Model file for the job. Use its own axes, mm. Coordinates: 2 decimals unless noted, no trailing zeros. Loops run counter-clockwise (first coordinate to the right, second up) from the corner with the lowest first, then second, coordinate; pieces in that order, holes last.
from build123d import *

# Parameters (mm, degrees)
SKETCH1_R           = 80
BOSS_EXTRUDE1_DEPTH = 20
SKETCH3_R           = 15
BOSS_EXTRUDE2_DEPTH = 15
CHAMFER1_SIZE       = 5
FILLET2_R           = 5
FILLET3_R           = 5
SKETCH4_R           = 5
CUT_EXTRUDE2_DEPTH  = 20


with BuildPart() as part:
    # Sketch1 → Boss-Extrude1 (new body)
    with BuildSketch(Plane(origin=(0, 0, 0), x_dir=(1, 0, 0), z_dir=(0, 1, 0))):
        with Locations(Location((-29.715512057, 28.347034528, 0), (0, 0, 270))):
            Circle(SKETCH1_R)
    extrude(amount=BOSS_EXTRUDE1_DEPTH)

    # Sketch3 → Boss-Extrude2 (add)
    with BuildSketch(Plane(origin=(0, 20, 0), x_dir=(1, 0, 0), z_dir=(0, 1, 0))):
        with Locations(Location((-29.715512057, 28.347034528, 0), (0, 0, 270))):
            Circle(SKETCH3_R)
    extrude(amount=BOSS_EXTRUDE2_DEPTH)

    # Chamfer1
    chamfer1_edges = [part.edges().sort_by_distance(p)[0] for p in [
        (-29.715512057, 35, -43.347034528),
    ]]
    chamfer(chamfer1_edges, length=CHAMFER1_SIZE)

    # Fillet2
    fillet2_edges = [part.edges().sort_by_distance(p)[0] for p in [
        (-29.715512057, 20, -108.347034528),
    ]]
    fillet(fillet2_edges, radius=FILLET2_R)

    # Fillet3
    fillet3_edges = [part.edges().sort_by_distance(p)[0] for p in [
        (-29.715512057, 0, -108.347034528),
    ]]
    fillet(fillet3_edges, radius=FILLET3_R)

    # Sketch4 → Cut-Extrude2 (cut)
    with BuildSketch(Plane(origin=(0, 20, 0), x_dir=(1, 0, 0), z_dir=(0, 1, 0))):
        with Locations(Location((-29.715512057, 77.081261822, 0), (0, 0, 270))):
            Circle(SKETCH4_R)
        with Locations(Location((-1.070251971, 67.773852617, 0), (0, 0, 270))):
            Circle(SKETCH4_R)
        with Locations(Location((16.633492378, 43.406738969, 0), (0, 0, 270))):
            Circle(SKETCH4_R)
        with Locations(Location((16.633492378, 13.287330086, 0), (0, 0, 270))):
            Circle(SKETCH4_R)
        with Locations(Location((-1.070251971, -11.079783561, 0), (0, 0, 270))):
            Circle(SKETCH4_R)
        with Locations(Location((-29.715512057, -20.387192767, 0), (0, 0, 270))):
            Circle(SKETCH4_R)
        with Locations(Location((-58.360772142, -11.079783561, 0), (0, 0, 270))):
            Circle(SKETCH4_R)
        with Locations(Location((-76.064516492, 13.287330086, 0), (0, 0, 270))):
            Circle(SKETCH4_R)
        with Locations(Location((-76.064516492, 43.406738969, 0), (0, 0, 270))):
            Circle(SKETCH4_R)
        with Locations(Location((-58.360772142, 67.773852617, 0), (0, 0, 270))):
            Circle(SKETCH4_R)
    extrude(amount=-CUT_EXTRUDE2_DEPTH, mode=Mode.SUBTRACT)


solid = part.part
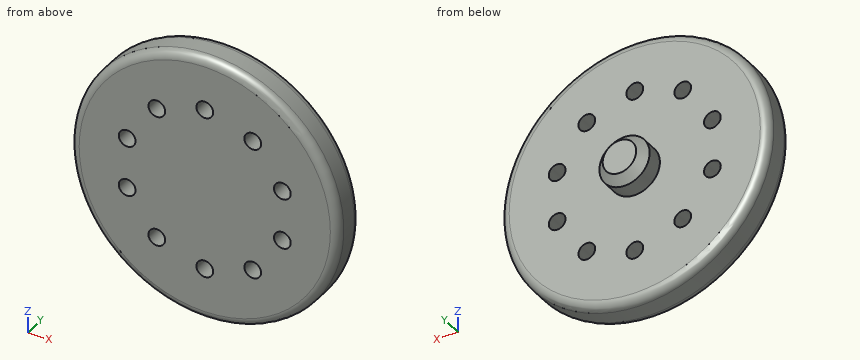
Q1. Flat gauge pins, fed straight in: P1, Ø8, axis at x = -78.5, y = 8, coming from the +Z side; P2, Ø6, axis at x = 5, y = 18, coming from the +Z side; P3, Ø12, axis at x = 31, y = 15, coming from the +Z side. Where does each tip first touch, or does it go through?
Answers:
P1: stops at z = 37.94
P2: stops at z = 44.68
P3: stops at z = 30.02
Q2. Drill centre lines: line 1 (Z direction, x = -59, y = 4.5); line 2 (Z direction, x = -5, y = 12); line 3 (Y direction, x = -73, z = -65). Where is each one in solid material? Low to high.
Answers:
line 1: z = -102.77 to -72.73, -62.81 to 6.12, 16.04 to 46.07
line 2: z = -104.43 to -70.87, -64.68 to 7.99, 14.17 to 47.74
line 3: y = 0 to 20
Q3. Slice it at C-C (y = 27.5). List the corners of the cut face in (x, z), and give its area (3 significant figures).
Answers:
outline: circle Ø30 at (-29.72, -28.35)
area: 707 mm2
Q4. Slice it at A-A (y = 17). Count the separate pieces of the cut face and the enclosed holes in it, and give its area (3 significant figures).
Answers:
separate pieces: 1
enclosed holes: 10
area: 19,100 mm2
